Autodesk Inventor part; units mm, degrees
ref_plane "dome work plane" through (56.8266, 25.4, -240.9792) normal (0.9733039, 0, 0.22952) x (0.22952, 0, -0.9733039)
ref_plane "door slot mirror" through (766.3795, 25.4, 180.7241) normal (0.22952, 0, -0.9733039) x (-0.9733039, 0, -0.22952)
ref_plane "YZ Plane" through (0, 0, 0) normal (1, 0, 0) x (0, 1, 0)
sketch "Sketch1" plane through (0, 0, 0) normal (0, 1, 0) x (-1, 0, 0)
  line L0 (707.6587, -429.7359) -> (319.9155, -763.615)
  line L1 (319.9155, -763.615) -> (-190.0245, -805.8191)
  line L2 (-190.0245, -805.8191) -> (-627.3817, -540.2278)
  line L3 (-627.3817, -540.2278) -> (-825.1003, -68.2877)
  line L4 (-825.1003, -68.2877) -> (-707.6587, 429.7359)
  line L5 (-707.6587, 429.7359) -> (-319.9155, 763.615)
  line L6 (-319.9155, 763.615) -> (190.0245, 805.8191)
  line L7 (190.0245, 805.8191) -> (627.3817, 540.2278)
  line L8 (627.3817, 540.2278) -> (825.1003, 68.2877)
  line L9 (825.1003, 68.2877) -> (707.6587, -429.7359)
  point P0 (0, 0)
  point P1 (0, 0)
  dimension "d0" = 1574.8
extrude "bace" add sketch "Sketch1" along normal blind 25.4
sketch "Sketch2" plane through (0, 25.4, 0) normal (0, 1, 0) x (1, 0, 0)
  line L0 (-319.9155, 763.615) -> (-707.6587, 429.7359)
  line L1 (-707.6587, 429.7359) -> (-319.9155, 763.615)
  line L2 (-319.9155, 763.615) -> (190.0245, 805.8191)
  line L3 (190.0245, 805.8191) -> (627.3817, 540.2278)
  line L4 (627.3817, 540.2278) -> (825.1003, 68.2877)
  line L5 (825.1003, 68.2877) -> (707.6587, -429.7359)
  line L6 (707.6587, -429.7359) -> (319.9155, -763.615)
  line L7 (319.9155, -763.615) -> (-190.0245, -805.8191)
  line L8 (-190.0245, -805.8191) -> (-627.3817, -540.2278)
  line L9 (-627.3817, -540.2278) -> (-825.1003, -68.2877)
  line L10 (-825.1003, -68.2877) -> (-707.6587, 429.7359)
  line L11 (-684.831, 415.8734) -> (-309.5957, 738.9822)
  line L12 (-309.5957, 738.9822) -> (183.8947, 779.825)
  line L13 (183.8947, 779.825) -> (607.1435, 522.8011)
  line L14 (607.1435, 522.8011) -> (798.4842, 66.0849)
  line L15 (798.4842, 66.0849) -> (684.831, -415.8734)
  line L16 (684.831, -415.8734) -> (309.5957, -738.9822)
  line L17 (309.5957, -738.9822) -> (-183.8947, -779.825)
  line L18 (-183.8947, -779.825) -> (-607.1435, -522.8011)
  line L19 (-607.1435, -522.8011) -> (-798.4842, -66.0849)
  line L20 (-798.4842, -66.0849) -> (-684.831, 415.8734)
  line L21 (-707.6587, 429.7359) -> (-825.1003, -68.2877)
  point P0 (0, 0)
  point P1 (0, 0)
  point P2 (0, 0)
  dimension "d4" = 25.4
extrude "bace wall" add sketch "Sketch2" along normal blind 508
sketch "Sketch3" plane through (0, 533.4, 0) normal (0, 1, 0) x (1, 0, 0)
  line L0 (-627.3817, -540.2278) -> (-825.1003, -68.2877)
  line L1 (-825.1003, -68.2877) -> (-707.6587, 429.7359)
  line L2 (-707.6587, 429.7359) -> (-319.9155, 763.615)
  line L3 (-319.9155, 763.615) -> (190.0245, 805.8191)
  line L4 (190.0245, 805.8191) -> (627.3817, 540.2278)
  line L5 (627.3817, 540.2278) -> (825.1003, 68.2877)
  line L6 (825.1003, 68.2877) -> (707.6587, -429.7359)
  line L7 (707.6587, -429.7359) -> (319.9155, -763.615)
  line L8 (319.9155, -763.615) -> (-190.0245, -805.8191)
  line L9 (-190.0245, -805.8191) -> (-627.3817, -540.2278)
  line L10 (-627.3817, -540.2278) -> (-825.1003, -68.2877)
  circle A0 centre (0, 0) radius 508
  point P0 (-798.4842, -66.0849)
  dimension "d28" = 1016
extrude "bace cieiling" add sketch "Sketch3" along normal blind 25.4
ref_plane "dome work plane" through (56.8266, 25.4, -240.9792) normal (0.9733039, 0, 0.22952) x (0.22952, 0, -0.9733039)
sketch "Sketch10" plane through (56.8266, 25.4, -240.9792) normal (0.9733039, 0, 0.22952) x (0.22952, 0, -0.9733039)
  line L0 (285.8112, 533.4) -> (260.4112, 533.4)
  line L1 (-755.5888, 533.4) -> (260.4112, 533.4)
  arc A0 (260.4112, 533.4) -> (-247.5888, 1041.4) centre (-247.5888, 533.4) ccw
  arc A1 (285.8112, 533.4) -> (-247.5888, 1066.8) centre (-247.5888, 533.4) ccw
  line L2 (-247.5888, 1066.8) -> (-247.5888, 1041.4)
  line L3 (-247.5888, 1041.4) -> (-247.5888, 533.4) construction
  point P0 (-247.5888, -25.4)
  dimension "d32" = 508
  dimension "d33" = 533.4
revolve "dome" add sketch "Sketch10" angle 360 about axis through (0, 1066.8, 0) along (0, -1, 0)
sketch "Sketch8" plane through (825.1003, 0, -68.2877) normal (0.9733039, 0, 0.22952) x (0.22952, 0, -0.9733039)
  line L0 (-255.8418, 25.4) -> (-205.0418, 25.4)
  line L1 (-205.0418, 25.4) -> (-205.0418, 194.7333)
  line L2 (-205.0418, 194.7333) -> (-255.8418, 194.7333)
  line L3 (-255.8418, 194.7333) -> (-255.8418, 25.4)
  line L4 (-255.8418, 25.4) -> (-306.6418, 25.4)
  line L5 (-306.6418, 25.4) -> (-306.6418, 194.7333)
  line L6 (-306.6418, 194.7333) -> (-255.8418, 194.7333)
  line L7 (-503.4306, 25.4) -> (-8.253, 25.4)
  point P0 (-255.8418, 0)
  point P1 (-255.8418, 25.4)
  dimension "d16" = 50.8
  dimension "d17" = 169.3333
extrude "door frame" cut sketch "Sketch8" against normal blind 25.4
sketch "Sketch7" plane through (825.1003, 0, -68.2877) normal (0.9733039, 0, 0.22952) x (0.22952, 0, -0.9733039)
  line L0 (-306.6418, 194.7333) -> (-205.0418, 194.7333)
  line L1 (-306.6418, 25.4) -> (-205.0418, 25.4)
  arc A0 (-198.4359, 0) -> (-313.6926, 0.2332) centre (-255.8418, 110.0667) ccw
  arc A1 (-306.6418, 194.7333) -> (-306.6418, 25.4) centre (-255.8418, 110.0667) ccw
  arc A2 (-205.0418, 25.4) -> (-205.0418, 194.7333) centre (-255.8418, 110.0667) ccw
  line L2 (-306.6418, 194.7333) -> (-205.0418, 194.7333)
  line L3 (-306.6418, 194.7333) -> (-306.6418, 25.4)
  line L4 (-313.6926, 0.2332) -> (-198.4359, 0)
  point P0 (-255.8418, 0)
  point P1 (-255.8418, 194.7333)
  point P2 (-306.6418, 110.0667)
  point P3 (-255.8418, 110.0667)
  point P4 (-256.0642, 0.1166)
  dimension "d14" = 169.3333
  dimension "d15" = 101.6
extrude "corridor connection" add sketch "Sketch7" along normal blind 25.4
sketch "Sketch9" plane through (729.998, 25.4, 224.3381) normal (0.22952, 0, -0.9733039) x (-0.9733039, 0, -0.22952)
  line L0 (-12.7, 169.3333) -> (-6.35, 169.3333)
  line L1 (-6.35, 169.3333) -> (-6.35, 0)
  line L2 (-6.35, 0) -> (-19.05, 0)
  line L3 (-19.05, 0) -> (-19.05, 169.3333)
  line L4 (-12.7, 169.3333) -> (-19.05, 169.3333)
  line L5 (-25.4, -25.4) -> (-25.4, 208.8041)
  point P0 (762, -25.4)
  point P1 (-25.4, -25.4)
  point P2 (-25.4, 169.3333)
  point P3 (0, 169.3333)
  point P4 (-25.4, 0)
  point P5 (0, 0)
  point P6 (-25.4, 169.3333)
  point P7 (-25.4, -25.1668)
  dimension "d22" = 6.35
  dimension "d23" = 12.7
  dimension "d24" = 169.3333
extrude "left door slot" cut sketch "Sketch9" against normal blind 50.8
ref_plane "door slot mirror" through (766.3795, 25.4, 180.7241) normal (0.22952, 0, -0.9733039) x (-0.9733039, 0, -0.22952)
mirror "Mirror1" about plane through (766.3795, 25.4, 180.7241) normal (0.22952, 0, -0.9733039) of "left door slot"
properties part number "dome"
Geometry check sheet. Reference: the model listing, model coordinates, mm. A direction names the side the tool comes from. Round coordinates to 2 decimals unless told otherwise and drop trailing zeros. Write each loop counter-clockwise with the first axis right and the second up, starting at its lowest first coordinate (ties: lowest second). Pieces come first, ordered by that corner, then holes. Notation, with made-up numbers: (-7.5, 24) - (5.5, 24) arc R25 cw to (5.5, 46) - close; hole circle Ø9 at (6.5, -30). An arc over 180 degrees is marked (long way). One line per item, written item: value.
1. Cross-section at A-A on z = 636.5. Record the boundary of the cut face in (x, y).
The answers:
outline: (-468.85, 0) - (467.54, 0) - (467.54, 558.8) - (-468.85, 558.8) - close; hole (-419.91, 25.4) - (428.61, 25.4) - (428.61, 533.4) - (-419.91, 533.4) - close
2. Depth check by flat-ended pin: pin 1 Ø10 at (x, y) = (-69, 356) entering from -Z; pin 2 Ø10 at (x, z) = (-314.5, -605) entering from +Y; pin 3 Ø1.5 at (y, z) = (854.5, 136) entering from +X. Enter the tip coordinate at first touch or a pass-through.
The answers:
pin 1: stops at z = -784.8
pin 2: stops at y = 558.8
pin 3: stops at x = 423.17
3. Scan lines: L1, parallel to Y at x = -190, z = 555; L2, parallel to Y at x = 337.5, z = -315; L3, parallel to X at y = 543.5, z = 0. Record each from-to range of solid material in increasing order.
The answers:
L1: y = 0 to 25.4, 533.4 to 558.8
L2: y = 0 to 25.4, 770.77 to 825.98
L3: x = -809 to -508, 508 to 809
4. Cross-section at C-C on y = 848. Record the boundary of the cut face in (x, z), and give its area (3 significant figures).
The answers:
outline: circle Ø896.39 at (0, 0); hole circle Ø835.29 at (0, 0)
area: 83,100 mm^2
5. Set-up check for faces 5 (the face through (790.968, 204.391, 187.118)), 6 (the face through (-66.3, 275.84, -759.12)), 7 (the face through (750.518, 108.881, 247.986)), 8 (the face through (782.395, 108.881, 112.809)): record each of +Z, -Z, +X, -X, +Y, -Y from which the full face is reachable in a straight line by a thin tool's end or side.
The answers:
face 5: +Z, +X, +Y, -Y
face 6: none
face 7: +X
face 8: +Z
6. Mould release check, pull along X, two halves, no side actions. Record for faces 1 (the face through (-767.2, 275.49, -177.24)), 2 (the face through (724.857, 275.488, -307.561)), 3 (the face through (-742.453, 275.844, -171.521)), 4 (the face through (777.565, 234.127, 187.85)): released by +X, released by -X, zero draft, split by the parting line, or undercut.
The answers:
face 1: released by -X
face 2: released by +X
face 3: undercut
face 4: undercut
7. Cross-section at B-B on x = 486. Record the boundary of the cut face in (y, z), and give its area (3 significant figures).
The answers:
outline: (0, -626.08) - (558.8, -626.08) - (558.8, -219.82) arc R219.82 ccw to (558.8, 219.82) - (558.8, 620.6) - (0, 620.6) - close; hole (25.4, -596.37) - (533.4, -596.37) - (533.4, -147.88) - (558.8, -147.88) arc R147.88 ccw to (558.8, 147.88) - (533.4, 147.88) - (533.4, 587.08) - (25.4, 587.08) - close
area: 129,000 mm^2
8. Cross-section at D-D on z = -255.5. Record the boundary of the cut face in (x, y), and give its area (3 significant figures).
The answers:
outline: (-748.75, 0) - (746.67, 0) - (746.67, 558.8) - (468.23, 558.8) arc R468.23 ccw to (-468.23, 558.8) - (-748.75, 558.8) - close; hole (-722.65, 25.4) - (719.13, 25.4) - (719.13, 533.4) - (439.07, 533.4) - (439.07, 558.8) arc R439.07 ccw to (-439.07, 558.8) - (-439.07, 533.4) - (-722.65, 533.4) - close
area: 122,000 mm^2
